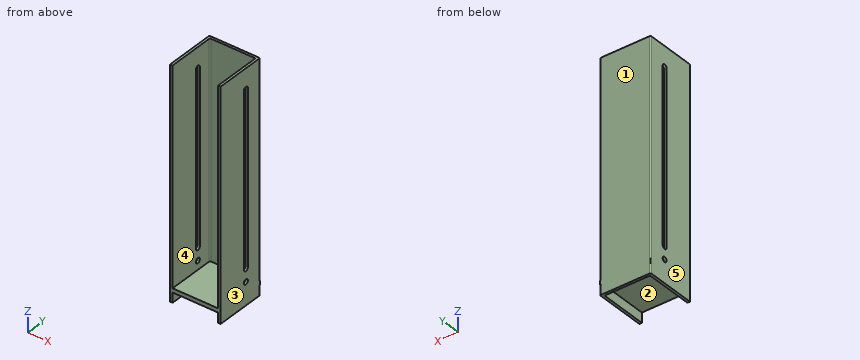
from build123d import *

# Parameters (mm, degrees)
F1_DEPTH = 225
F3_DEPTH = 60
F2_W     = 100
F2_H     = 8
F4_DEPTH = 50


with BuildPart() as f1:
    # F0 (on Top) → F1 (new body, symmetric)
    with BuildSketch(Plane.XY):
        with BuildLine():
            Line((-50, 28.660538), (-50, -69.339462))
            Line((-50, -69.339462), (-45, -69.339462))
            Line((-45, -69.339462), (-45, 23.660538))
            ThreePointArc((-45, 23.660538), (-44.414214, 25.074752), (-43, 25.660538))
            Line((-43, 25.660538), (43, 25.660538))
            ThreePointArc((43, 25.660538), (44.414214, 25.074752), (45, 23.660538))
            Line((45, 23.660538), (45, -69.339462))
            Line((45, -69.339462), (50, -69.339462))
            Line((50, -69.339462), (50, 28.660538))
            ThreePointArc((50, 28.660538), (49.414214, 30.074752), (48, 30.660538))
            Line((48, 30.660538), (-48, 30.660538))
            ThreePointArc((-48, 30.660538), (-49.414214, 30.074752), (-50, 28.660538))
        make_face()
    extrude(amount=F1_DEPTH, both=True)

    # F2 (on Right) → F3 (cut, symmetric)
    with BuildSketch(Plane.YZ):
        with BuildLine():
            Line((0, -155), (0, 185))
            ThreePointArc((0, 185), (-1.464466, 188.535534), (-5, 190))
            ThreePointArc((-5, 190), (-8.535534, 188.535534), (-10, 185))
            Line((-10, 185), (-10, -155))
            ThreePointArc((-10, -155), (-8.535534, -158.535534), (-5, -160))
            ThreePointArc((-5, -160), (-1.464466, -158.535534), (0, -155))
        make_face()
        with BuildLine():
            ThreePointArc((0, -180), (-1.464466, -176.464466), (-5, -175))
            ThreePointArc((-5, -175), (-8.535534, -183.535534), (0, -180))
        make_face()
    extrude(amount=F3_DEPTH, both=True, mode=Mode.SUBTRACT)

    # F2 (on Right) → F4 (join, symmetric)
    with BuildSketch(Plane.YZ):
        with Locations((-19.339462, -201.432384)):
            Rectangle(F2_W, F2_H)
    extrude(amount=F4_DEPTH, both=True)


solid = f1.part
Here's how the part is built. I have some questions about the finished solid (model axes, mm). Face numbers are marked on the shaded views. A direction names the side the tool comes from. Give positions to 0.01 mm unless a question says otherwise; leave off trailing zeros. Write each loop counter-clockwise with the first axis right and the second up, starting at its lowest first coordinate (ties: lowest second). Pieces come first, ordered by that corner, then holes. Notation, with made-up numbers: (71.5, -37) -> (117.5, -37) arc R22 cw to (117.5, -22) -> close; hole circle Ø5 at (50, 29.5). An arc over 180 degrees is marked (long way). Use one line per item in the form item = value. Start each with the question number.
1. Imagine slicing it at C-C on y = -43. List the corners of the cut face in (x, z) for me, plus the area to 3 significant figures.
2. Will these pins go through, and if not, where does the flat tip stop? pin 1 Ø3 at (x, y) = (-9.5, -53.5) entering from -Z; pin 2 Ø6 at (x, z) = (21.5, 154) entering from -Y; pin 3 Ø8 at (y, z) = (-5, -180) entering from +X; pin 4 Ø5 at (x, y) = (-10.5, -3) entering from +Z.
3. Imagine slicing it at A-A on z = 14. List the corners of the cut face in (x, y) for me.
4. On a 3-axis mill with a long thin cutter (end or side, diameter ignored), from which of +Z, -Z, +X, -X, +Y, -Y can I reach the whole of each face in a straight line? I mean the marked faces 4 and 5. Say none if no direction works.
5. Thinking about a two-plate mould opening in X: for the marked faces 1, 2 and 3, which applies, +X half, -X half, draft (parallel to the pull), parting line (faces both ways), or undercut?
6. If I drill on L1, parallel to Z at x = -46.2, y = -5; L2, parallel to X at y = -50, z = 134; L3, parallel to Y at x = -47, z = -180, over which ranges is the centre line in solid material (lowest first)?
7. Imagine slicing it at B-B on x = -10. List the corners of the cut face in (y, z) for me, plus the area to 3 significant figures.
Entries:
q1.outline = (-50, -225) -> (-45, -225) -> (-45, -205.43) -> (45, -205.43) -> (45, -225) -> (50, -225) -> (50, 225) -> (45, 225) -> (45, -197.43) -> (-45, -197.43) -> (-45, 225) -> (-50, 225) -> close
q1.area = 5,220 mm²
q2.pin_1 = -205.43
q2.pin_2 = 25.66
q2.pin_3 = through
q2.pin_4 = -197.43
q3.outline = (-50, -69.34) -> (-45, -69.34) -> (-45, -10) -> (-50, -10) -> close; (-50, 0) -> (-45, 0) -> (-45, 23.66) arc R2 cw to (-43, 25.66) -> (43, 25.66) arc R2 cw to (45, 23.66) -> (45, 0) -> (50, 0) -> (50, 28.66) arc R2 ccw to (48, 30.66) -> (-48, 30.66) arc R2 ccw to (-50, 28.66) -> close; (45, -69.34) -> (50, -69.34) -> (50, -10) -> (45, -10) -> close
q4.face_4 = +Z, -Y
q4.face_5 = +Z, -Z, -X, +Y, -Y
q5.face_1 = draft
q5.face_2 = undercut
q5.face_3 = +X half
q6.L1 = -225 to -185, -175 to -160, 190 to 225
q6.L2 = -50 to -45, 45 to 50
q6.L3 = -69.34 to -10, 0 to 30.66
q7.outline = (-69.34, -205.43) -> (25.66, -205.43) -> (25.66, -225) -> (30.66, -225) -> (30.66, 225) -> (25.66, 225) -> (25.66, -197.43) -> (-69.34, -197.43) -> close
q7.area = 3,010 mm²
